Can you work these out from the drawing? Everything is in mm from the part's minimum corner. A direction names the side the tool comes from. Round coordinates to 2 decimals unless told otherwise and drop trailing zeros. Loops run counter-clockwise (first coordinate to the right, second up) from the corner with the lowest first, then second, coordinate; pieces in that order, holes last. Notation, with made-up numbers: (87, 73) - (114, 73) arc R26 cw to (114, 95) - close; hole circle Ø1 at (4, 24.5). An arc over 180 degrees is marked (long way). Answer as a JSON object with one key per item and string values. Group by question number.
1) I want a section at A-A, the plane x = 7.5. Please give me the cut outline in (y, z), then the cut area to 4 significant figures.
2) If we mould it in two halves opening along X, with no side actions, what happens to the marked faces 3, 4 and 5? For each: pulls with the +X half, pulls with the -X half, needs draft (parallel to the pull), parting line crosses it, or undercut.
3) I want a section at D-D, the plane x = 5.75. Please give me the cut outline in (y, z).
4) I want a section at C-C, the plane y = 19.5. Please give me the cut outline in (x, z), then the cut area to 3 significant figures.
5) I want a section at B-B, the plane z = 1. Please give me the cut outline in (x, y), then the cut area to 3 significant figures.
6) Which directions (+Z, -Z, +X, -X, +Y, -Y) give clear straight access to the entire face, cutting with the end or side of a thin tool? Please do the marked faces 1 and 2.
7) If I drill on line 1 along Y through (x, z) = (7.5, 1.25); line 2 along X through (y, z) = (20, 2.85); line 3 along Z through (x, y) = (2.5, 2), over which ranges is the centre line in solid material (lowest first)? Write a range as [from, to].
8) Will these pins go through, and if not, where does the flat tip stop? P1, Ø4, axis at x = 7.5, y = 20, coming from the +Z side; P2, Ø2, axis at x = 10, z = 2.5, coming from the +Y side; P3, Ø2, axis at x = 4.5, z = 2, coming from the +Y side; P4, Ø8, axis at x = 7, y = 6.5, coming from the -Z side.
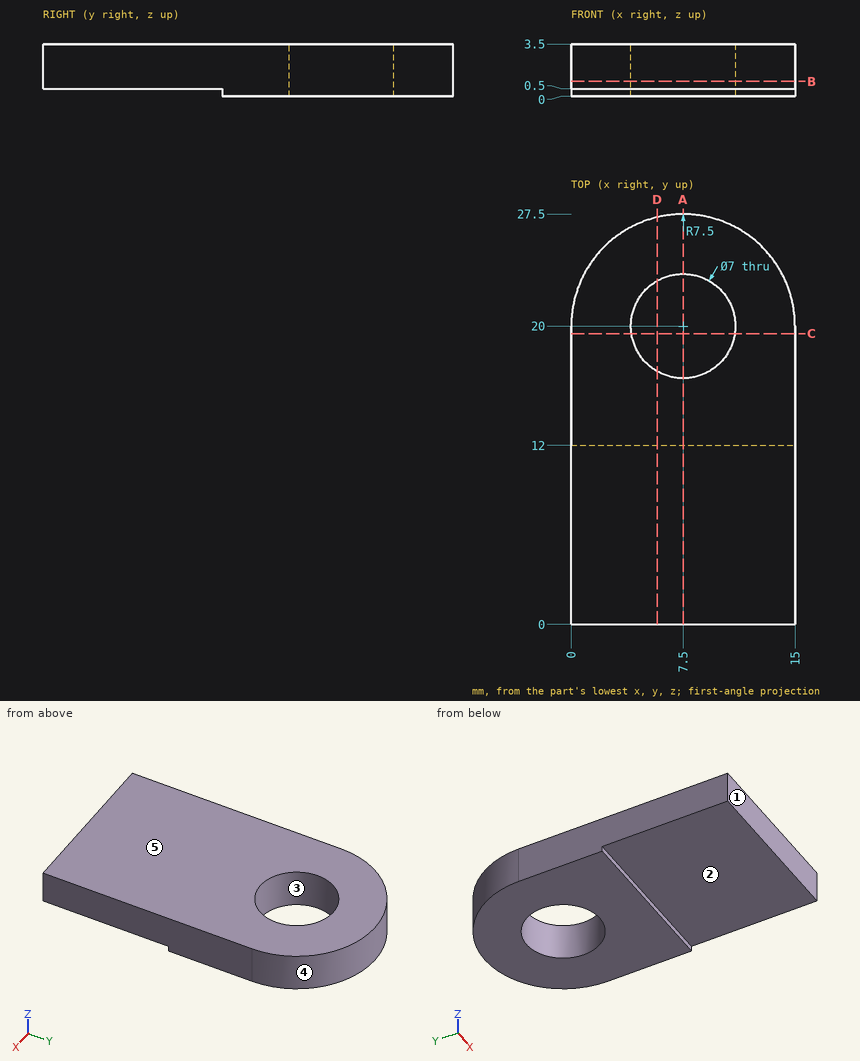
Outcome:
{
 "1": {"outline": "(0, 0.5) - (12, 0.5) - (12, 0) - (16.5, 0) - (16.5, 3.5) - (0, 3.5) - close; (23.5, 0) - (27.5, 0) - (27.5, 3.5) - (23.5, 3.5) - close", "area": "65.75 mm^2"},
 "2": {"face 3": "undercut", "face 4": "parting line crosses it", "face 5": "needs draft"},
 "3": {"outline": "(0, 0.5) - (12, 0.5) - (12, 0) - (16.97, 0) - (16.97, 3.5) - (0, 3.5) - close; (23.03, 0) - (27.29, 0) - (27.29, 3.5) - (23.03, 3.5) - close"},
 "4": {"outline": "(0, 0) - (4.04, 0) - (4.04, 3.5) - (0, 3.5) - close; (10.96, 0) - (15, 0) - (15, 3.5) - (10.96, 3.5) - close", "area": "28.3 mm^2"},
 "5": {"outline": "(0, 0) - (15, 0) - (15, 20) arc R7.5 ccw to (0, 20) - close; hole circle Ø7 at (7.5, 20)", "area": "350 mm^2"},
 "6": {"face 1": "+Z, -Z, +X, -X, -Y", "face 2": "-Z, +X, -X, -Y"},
 "7": {"line 1": "[0, 16.5], [23.5, 27.5]", "line 2": "[0, 4], [11, 15]", "line 3": "[0.5, 3.5]"},
 "8": {"P1": "through", "P2": "y = 27.35", "P3": "y = 27.23", "P4": "z = 0.5"}
}
